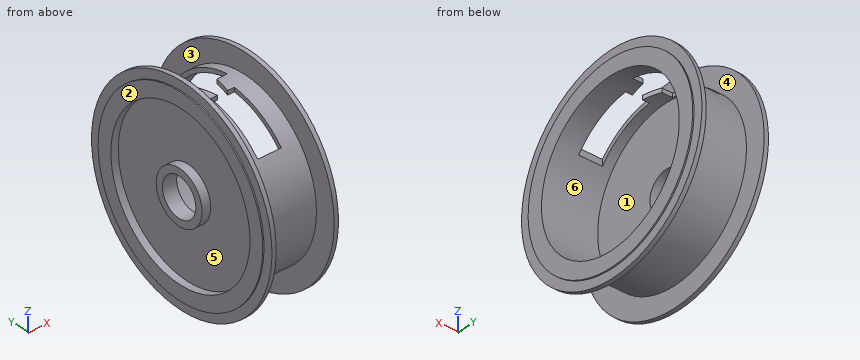
from build123d import *

# Parameters (mm, degrees)
KES_EKSTR_ZYON1_DEPTH = 38.65222437


with BuildPart() as part:
    # Çizim1 → Döndür1 (revolve)
    with BuildSketch(Plane.XY, mode=Mode.PRIVATE) as d_nd_r1_sk:
        Polygon((0.3, 18.5), (0.3, 21.9), (0.6, 21.9), (0.6, 24), (1.6, 24), (1.6, 19.3), (15, 19.3), (15, 24), (16, 24), (16, 21.9), (16.3, 21.9), (16.3, 18.35), (3.3, 18.35), (3.3, 4.45), (0, 4.45), (0, 6.1), (2, 6.1), (2, 18.5), align=None)
    revolve(d_nd_r1_sk.sketch.rotate(Axis((-5.366453406, 0, 0), (1, 0, 0)), 90), axis=Axis((-5.366453406, 0, 0), (1, 0, 0)))

    # Çizim2 → Kes-Ekstrüzyon1 (cut, through all)
    with BuildSketch(Plane.XY):
        Polygon((12.925, 14.5), (3.675, 14.5), (3.675, 2), (6.15, 2), (7.15, -2), (5.55, -2), (5.55, -14.5), (11.05, -14.5), (11.05, -2), (9.45, -2), (10.45, 2), (12.925, 2), align=None)
    extrude(amount=KES_EKSTR_ZYON1_DEPTH, mode=Mode.SUBTRACT)


solid = part.part
Geometry check sheet. Reference: the model listing, model coordinates, mm. Face numbers are marked on the shaded views. A direction names the side the tool comes from. Coordinates: 2 decimals unless noted, no trailing zeros. Order: outer loops, then holes, each group sorted by start corner. A loop starts at its lowest first (then second) coordinate and runs counter-clockwise, first axis right, second up. Notation, with made-up numbers: M 26,2.5 L 61,2.5 A31 cw 61,40.5 Z; hole C 31.5,-13 d10. An arc over 180 degrees is marked long. Use CSV: the item, a comma, the result in double quotes.
Item 1: Gauge pin test, flat ends, axial feed: pin 1 Ø2.5 at (y, z) = (-5.5, 16.5) entering from -X; pin 2 Ø1 at (x, z) = (5.5, -2) entering from -Y; pin 3 Ø6 at (x, z) = (14.5, -17.5) entering from -Y. Record the tip position at first contact, or that the pin passes through.
Returned:
pin 1,"stops at x = 0.3"
pin 2,"stops at y = -19.24"
pin 3,"stops at y = -19.09"
Item 2: Cross-section at B-B on z = -20. Record the cut outline in (x, y).
Returned:
outline,"M 0.3,-8.92 L 0.6,-8.92 L 0.6,-13.27 L 1.6,-13.27 L 1.6,13.27 L 0.6,13.27 L 0.6,8.92 L 0.3,8.92 Z; M 15,-13.27 L 16,-13.27 L 16,-8.92 L 16.3,-8.92 L 16.3,8.92 L 16,8.92 L 16,13.27 L 15,13.27 Z"
Item 3: Cross-section at C-C on y = 0. Give the number of separate pieces and of enclosed holes in the cut face, then the cut area to 3 significant figures.
Returned:
separate pieces,"3"
enclosed holes,"0"
area,"91.4 mm2"
Item 4: Mould release check, pull along X, two halves, no side actions. Record for the marked faces 1, 2 and 3: pulls with the +X half, pulls with the -X half, needs draft (parallel to the pull), parting line crosses it, or undercut.
Returned:
face 1,"pulls with the +X half"
face 2,"pulls with the -X half"
face 3,"undercut"
Item 5: Tool access check on the marked faces 4, 5 and 6. Record the directions out of +Z, -Z, +X, -X, +Y, -Y that give a thin tool (end or side, any length) a straight path to the whole face; none if there is none.
Returned:
face 4,"none"
face 5,"-X"
face 6,"+X"
Item 6: Thickness scan on line 1 along Y through (x, z) = (1.7, 0); line 2 along X through (y, z) = (17.5, -15.5); line 3 along X through (y, z) = (19.5, 5). Record the ranges inside material, lowest first.
Returned:
line 1,"y = -19.3 to -18.5, -6.1 to -4.45, 4.45 to 6.1, 18.5 to 19.3"
line 2,"x = 0.6 to 1.6, 15 to 16"
line 3,"x = 0.3 to 1.6, 15 to 16.3"
